Input: part model. Units: mm. Frame: model coordinates. A direction names the side the tool comes from. Give positions to 0.01 mm unless a question says otherwise; leave off trailing zeros. Order: outer loops, then holes, each group sorted by start corner. A loop starts at its lowest first (then second) coordinate and runs counter-clockwise, first axis right, second up. Notation, with made-up numbers: M 33.25,85 L 44.25,85 A16 cw 44.25,114 Z; hole C -20,-13 d2. An arc over 180 degrees is marked long. Use a Markdown table: item, result.
from build123d import *

# Parameters (mm, degrees)
F0_W     = 127
F0_H     = 50.8
F1_DEPTH = 25.4
F3_DEPTH = 635
F4_W     = 127
F4_H     = 25.4
F5_DEPTH = 254


with BuildPart() as f1:
    # F0 (on Top) → F1 (new body)
    with BuildSketch(Plane.XY):
        Polygon((1.767107, -22.436125), (1.767107, 28.363875), (-101.6, 0), align=None)
        Polygon((230.367107, 0), (128.767107, 28.363875), (128.767107, -22.436125), align=None)
        with Locations((65.267107, 2.963875)):
            Rectangle(F0_W, F0_H)
    extrude(amount=F1_DEPTH)

    # F2 (on face) → F3 (join)
    with BuildSketch(Plane.XY.offset(25.4)):
        Polygon((179.567107, 0), (-50.8, 0), (65.267107, -12.7), align=None)
        Polygon((65.267107, 12.7), (-50.8, 0), (179.567107, 0), align=None)
    extrude(amount=F3_DEPTH)

    # F4 (on face) → F5 (join)
    with BuildSketch(Plane(origin=(0, 0, 0), x_dir=(1, 0, 0), z_dir=(0, 0, -1))):
        with Locations((65.267107, -2.963875)):
            Rectangle(F4_W, F4_H)
    extrude(amount=F5_DEPTH)


solid = f1.part
1) First-contact query: pin 1 Ø6 at (x, z) = (127.5, 37) entering from +Y; pin 2 Ø3 at (x, z) = (-20.5, 436.5) entering from +Y; pin 3 Ø10 at (y, z) = (11.5, -129) entering from -X. Flat tips, straight axial feed; report the tip coordinate or a pass-through.
Response values:
| item | result |
|---|---|
| pin 1 | stops at y = 6.12 |
| pin 2 | stops at y = 3.48 |
| pin 3 | stops at x = 1.77 |
2) Cut plane C-C on x = 158. Return loops of the section in (y, z), and give its area (3 significant figures).
Response values:
| item | result |
|---|---|
| outline | M -15.98,0 L 20.2,0 L 20.2,25.4 L 2.4,25.4 L 2.4,660.4 L -2.4,660.4 L -2.4,25.4 L -15.98,25.4 Z |
| area | 3,960 mm² |
3) Cut plane D-D on x = 90. Return loops of the section in (y, z).
Response values:
| item | result |
|---|---|
| outline | M -22.44,0 L -9.74,0 L -9.74,-254 L 15.66,-254 L 15.66,0 L 28.36,0 L 28.36,25.4 L 9.95,25.4 L 9.95,660.4 L -9.95,660.4 L -9.95,25.4 L -22.44,25.4 Z |
4) Reachability of faces 1 (the face through (64, -9.736, -125)), 2 (the face through (128.767, 3, -125)), 3 (the face through (62, 15, 25.4)) from +Z, -Z, +X, -X, +Y, -Y: full face, straight path, thin tool, end or side. Return the list, or none.
Response values:
| item | result |
|---|---|
| face 1 | -Z, +X, -X, -Y |
| face 2 | -Z, +X, +Y, -Y |
| face 3 | +Z |
5) Material intervals for line 1 (Z direction, x = 178.5, y = 10.5); line 2 (X direction, y = -1, z = -85); line 3 (Z direction, x = 59.5, y = 14), sorted ascending. Write a range as from..to.
Response values:
| item | result |
|---|---|
| line 1 | z = 0..25.4 |
| line 2 | x = 1.77..128.77 |
| line 3 | z = -254..25.4 |
6) Cut plane A-A on x = 37.5. Return loops of the section in (y, z), and give its area (3 significant figures).
Response values:
| item | result |
|---|---|
| outline | M -22.44,0 L -9.74,0 L -9.74,-254 L 15.66,-254 L 15.66,0 L 28.36,0 L 28.36,25.4 L 9.66,25.4 L 9.66,660.4 L -9.66,660.4 L -9.66,25.4 L -22.44,25.4 Z |
| area | 20,000 mm² |
7) Cut plane B-B on z = 401. Return loops of the section in (x, y), and give its area (3 significant figures).
Response values:
| item | result |
|---|---|
| outline | M -50.8,0 L 65.27,-12.7 L 179.57,0 L 65.27,12.7 Z |
| area | 2,930 mm² |
